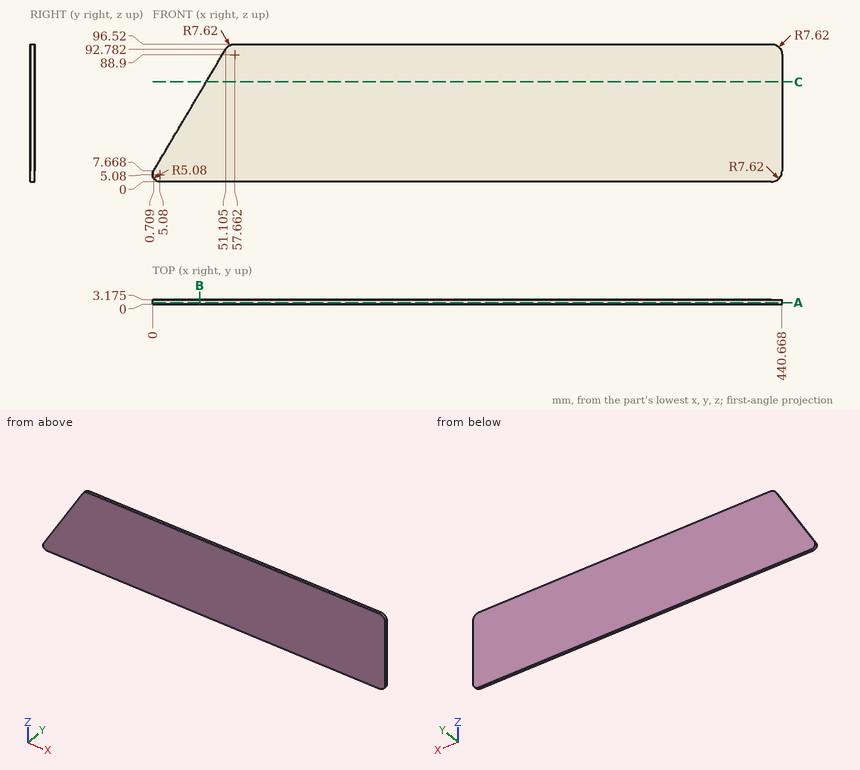
Verification items for this drawing (mm, ordinates from the low corner). Round coordinates to 2 decimals unless told otherwise and drop trailing zeros. Loops run counter-clockwise (first coordinate to the right, second up) from the corner with the lowest first, then second, coordinate; pieces in that order, holes last. Notation, with made-up numbers: M 52.25,10.25 L 67.25,10.25 A26 cw 67.25,48.25 Z; hole C 73.5,-39 d7. An arc over 180 degrees is marked long. Answer as a JSON object with one key per item and string values.
1. Scan lines: line 1 (X direction, y = 2.9, z = 51) (1 decimal); line 2 (X direction, y = 1.55, z = 64). Record each from-to range of solid material in increasing order.
Reply:
{"line 1": "x = 26.4 to 440.7", "line 2": "x = 34.06 to 440.67"}
2. Section check B-B (x = 33). Record the boundary of the cut face in (y, z) (1 decimal).
Reply:
{"outline": "M 0,0 L 3.2,0 L 3.2,62.2 L 0,62.2 Z"}
3. Section check A-A (y = 1.2). Record the boundary of the cut face in (x, z) (1 decimal), plus the area to 3 significant figures.
Reply:
{"outline": "M 0.7,7.7 A5.1 ccw 5.1,0 L 433,0 A7.6 ccw 440.7,7.6 L 440.7,88.9 A7.6 ccw 433,96.5 L 57.7,96.5 A7.6 ccw 51.1,92.8 Z", "area": "40,100 mm²"}
4. Section check C-C (z = 70). Record the boundary of the cut face in (x, y) (1 decimal), plus the area to 3 significant figures.
Reply:
{"outline": "M 37.6,0 L 440.7,0 L 440.7,3.2 L 37.6,3.2 Z", "area": "1,280 mm²"}
